Source: CAD feature listing. Evaluate the final solid. Frame: model axes, mm. A direction names the side the tool comes from. Give positions to 0.01 mm unless a question says otherwise; leave off trailing zeros. Order: outer loops, then holes, each group sorted by start corner. A loop starts at its lowest first (then second) coordinate and runs counter-clockwise, first axis right, second up.
from build123d import *

# Parameters (mm, degrees)
SKETCH1_R              = 3
SKETCH1_R_2            = 1.25
SKETCH1_R_3            = 1.5
SKETCH1_R_4            = 0.9
BOSS_EXTRUDE1_DEPTH    = 3
FILLET1_R              = 5
FILLET2_R              = 1
CUT_EXTRUDE1_DEPTH     = 100.949987494
SKETCH4_W              = 140
SKETCH4_H              = 3
BOSS_EXTRUDE2_DEPTH    = 20.5
FILLET4_R              = 3
CONVERT_SOLID1_START   = -65
CONVERT_SOLID1_DEPTH   = 140
CONVERT_SOLID1_2_DEPTH = 140
SKETCH9_R              = 3.4
CUT_EXTRUDE3_DEPTH     = 119.836021475


# Read off the part's stored shape, not the designer's step: Convert-Solid1
with BuildPart() as part:
    # Sketch1 → Boss-Extrude1 (new body)
    with BuildSketch(Plane(origin=(0, 0, 0), x_dir=(0, 0, -1), z_dir=(1, 0, 0))):
        with BuildLine():
            Line((0, 5), (65, 5))
            Line((65, 5), (65, 15))
            Line((65, 15), (-35, 15))
            Line((-35, 15), (-65.988977704, -10.781451876))
            ThreePointArc((-65.988977704, -10.781451876), (-72.635419618, -19.386905319), (-75, -30))
            Line((-75, -30), (-75, -66))
            Line((-75, -66), (65, -66))
            Line((65, -66), (65, -44))
            Line((65, -44), (0, -44))
            Line((0, -44), (0, 5))
        make_face()
        with Locations((-50, -30)):
            Circle(SKETCH1_R, mode=Mode.SUBTRACT)
        with Locations((55, 10)):
            Circle(SKETCH1_R_2, mode=Mode.SUBTRACT)
        with Locations((25, 10)):
            Circle(SKETCH1_R_2, mode=Mode.SUBTRACT)
        with Locations((-33.192050804, 10)):
            Circle(SKETCH1_R_2, mode=Mode.SUBTRACT)
        with Locations((-70, -30)):
            Circle(SKETCH1_R_2, mode=Mode.SUBTRACT)
        with Locations((-10, -50)):
            Circle(SKETCH1_R_2, mode=Mode.SUBTRACT)
        with Locations((-25, 4)):
            Circle(SKETCH1_R_3, mode=Mode.SUBTRACT)
        with Locations((-15, 4)):
            Circle(SKETCH1_R_3, mode=Mode.SUBTRACT)
        with Locations((-22, -14)):
            Circle(SKETCH1_R_4, mode=Mode.SUBTRACT)
        with Locations((-28.5, -14)):
            Circle(SKETCH1_R_4, mode=Mode.SUBTRACT)
    extrude(amount=BOSS_EXTRUDE1_DEPTH)

    # Fillet1
    fillet1_edges = [part.edges().sort_by_distance(p)[0] for p in [
        (1.5, 15, 35),
        (1.5, 15, -65),
    ]]
    fillet(fillet1_edges, radius=FILLET1_R)

    # Fillet2
    fillet2_edges = [part.edges().sort_by_distance(p)[0] for p in [
        (1.5, 5, -65),
        (1.5, -44, -65),
    ]]
    fillet(fillet2_edges, radius=FILLET2_R)

    # Sketch2 → Cut-Extrude1 (cut, through all)
    with BuildSketch(Plane(origin=(3, 0, 0), x_dir=(0, 0, -1), z_dir=(1, 0, 0))):
        with BuildLine():
            Line((-53.319244679, -40.106902918), (-53.373768913, -41.355713195))
            ThreePointArc((-53.373768913, -41.355713195), (-54.416436522, -42.31114203), (-55.371865356, -41.268474421))
            Line((-55.371865356, -41.268474421), (-55.317341122, -40.019664144))
            ThreePointArc((-55.317341122, -40.019664144), (-54.274673513, -39.06423531), (-53.319244679, -40.106902918))
        make_face()
        with BuildLine():
            Line((-55.80805923, -51.258956637), (-55.753534996, -50.01014636))
            ThreePointArc((-55.753534996, -50.01014636), (-54.710867387, -49.054717525), (-53.755438553, -50.097385134))
            Line((-53.755438553, -50.097385134), (-53.809962787, -51.346195411))
            ThreePointArc((-53.809962787, -51.346195411), (-54.852630396, -52.301624245), (-55.80805923, -51.258956637))
        make_face()
    extrude(amount=-CUT_EXTRUDE1_DEPTH, mode=Mode.SUBTRACT)

    # Sketch4 → Boss-Extrude2 (add)
    with BuildSketch(Plane.ZY):
        with Locations((5, -64.5)):
            Rectangle(SKETCH4_W, SKETCH4_H)
    extrude(amount=BOSS_EXTRUDE2_DEPTH)

    # Fillet4
    fillet4_edges = [part.edges().sort_by_distance(p)[0] for p in [
        (1.5, -44, 0),
    ]]
    fillet(fillet4_edges, radius=FILLET4_R)

    # Mirror1: part across plane


with BuildPart() as part_1:
    add(part.part)
    add(part.part.mirror(Plane(origin=(-20.5, 0, 0), x_dir=(0, 0, 1), z_dir=(1, 0, 0))))

    # Convert-Solid1 outline → Convert-Solid1 (cut)
    with BuildSketch(Plane.XY.offset(CONVERT_SOLID1_START)):
        with BuildLine():
            ThreePointArc((3, -59), (0.949747468, -63.949747468), (-4, -66))
            Line((-4, -66), (3, -66))
            Line((3, -66), (3, -59))
        make_face()
        with BuildLine():
            Line((-44, -66), (-37, -66))
            ThreePointArc((-37, -66), (-41.949747468, -63.949747468), (-44, -59))
            Line((-44, -59), (-44, -66))
        make_face()
    extrude(amount=CONVERT_SOLID1_DEPTH, mode=Mode.SUBTRACT)

    # Convert-Solid1 2 outline → Convert-Solid1 2 (add)
    with BuildSketch(Plane.XY.offset(CONVERT_SOLID1_START)):
        with BuildLine():
            Line((-41, -63), (-37, -63))
            ThreePointArc((-37, -63), (-39.828427125, -61.828427125), (-41, -59))
            Line((-41, -59), (-41, -63))
        make_face()
        with BuildLine():
            ThreePointArc((0, -59), (-1.171572875, -61.828427125), (-4, -63))
            Line((-4, -63), (0, -63))
            Line((0, -63), (0, -59))
        make_face()
    extrude(amount=CONVERT_SOLID1_2_DEPTH)

    # Sketch9 → Cut-Extrude3 (cut, through all)
    with BuildSketch(Plane.XZ.offset(66)):
        with Locations(Location((-20.5, -55, 0), (0, 0, 270))):
            Circle(SKETCH9_R)
    extrude(amount=-CUT_EXTRUDE3_DEPTH, mode=Mode.SUBTRACT)


solid = part_1.part
(1) Section C-C, the plane y = -18. Return loops of the section in (x, z).
(2) Section B-B, the plane z = 25. Return loops of the section in (x, y).
(3) Section A-A, the plane x = -20.5. Return loops of the section in (y, z).
(4) Pin query (flat end, axial travel): pin 1 Ø10 at (y, z) = (2, -28) entering from +X; pin 2 Ø3.5 at (x, y) = (-42, -22) entering from -Z. Return the tip coordinate at first contact, or that it passes through.
(5) Section D-D, the plane z = 60. Return loops of the section in (x, y).
(6) Draft query along Y for faces 4 (the cylindrical face through (-42, -30, 53)), 5 (the cylindrical face through (-39.797, -61.859, 4.02)), 6 (the cylindrical face through (1, -30, 53)), 7 (the flat face through (-41, -30, 22)). Return one class per face: +Y half, -Y half, draft (parallel to the pull), parting line (faces both ways), or undercut.
(7) Line query: line 1 along X through (y, z) = (-59.5, 15); line 2 along Y through (x, z) = (-42.2, -25); line 3 along Y through (x, z) = (-22, -27.5). Output: solid intervals per line, ascending.
(8) Access query for faces 1 (the flat face through (-21, -63, 4)), 2 (the flat face through (-42, 5, -32)), 3 (the flat face through (-42, 8, -65)). Directions: +Z, -Z, +X, -X, +Y, -Y. A direction counts if a zero-diameter tool reaches every point of the face in a straight line with its end or side. Return the directions, or none.
Checks:
1. outline: (-44, 0) - (-41, 0) - (-41, 71.93) - (-44, 71.93) - close; (0, 0) - (3, 0) - (3, 71.93) - (0, 71.93) - close
2. outline: (-44, -59) arc R7 ccw to (-37, -66) - (-4, -66) arc R7 ccw to (3, -59) - (3, 2.5) - (0, 2.5) - (0, -59) arc R4 cw to (-4, -63) - (-37, -63) arc R4 cw to (-41, -59) - (-41, 2.5) - (-44, 2.5) - close; (-44, 5.5) - (-41, 5.5) - (-41, 15) - (-44, 15) - close; (0, 5.5) - (3, 5.5) - (3, 15) - (0, 15) - close
3. outline: (-66, -65) - (-63, -65) - (-63, -58.4) - (-66, -58.4) - close; (-66, -51.6) - (-63, -51.6) - (-63, 75) - (-66, 75) - close
4. pin 1: stops at x = 3
4. pin 2: stops at z = 0
5. outline: (-44, -59) arc R7 ccw to (-37, -66) - (-4, -66) arc R7 ccw to (3, -59) - (3, -5.8) - (0, -5.8) - (0, -59) arc R4 cw to (-4, -63) - (-37, -63) arc R4 cw to (-41, -59) - (-41, -5.8) - (-44, -5.8) - close
6. face 4: undercut
6. face 5: +Y half
6. face 6: undercut
6. face 7: draft
7. line 1: x = -43.98 to -40.97, -0.03 to 2.98
7. line 2: y = -63.69 to -44, 5 to 8.75, 11.25 to 15
7. line 3: y = -66 to -63
8. face 1: +Z, -Z, +Y
8. face 2: -Z, +X, -X
8. face 3: -Z, +X, -X, +Y, -Y
